CAD build for the part. Positions are in the model's coordinates, mm. Give positions to 0.01 mm unless a question says otherwise; leave off trailing zeros. Loops run counter-clockwise (first coordinate to the right, second up) from the corner with the lowest first, then second, coordinate; pieces in that order, holes last.
```python
from build123d import *

# Parameters (mm, degrees)
F0_R     = 15.875
F0_R_2   = 9.525
F1_DEPTH = 25.4
F2_DEPTH = 25.4


with BuildPart() as f1:
    # F0 (on Top) → F1 (new body)
    with BuildSketch(Plane.XY):
        with BuildLine():
            ThreePointArc((5.357812, -28.068211), (22.018516, -18.21306), (28.575, 0))
            ThreePointArc((28.575, 0), (22.018516, 18.21306), (5.357812, 28.068211))
            ThreePointArc((5.357812, 28.068211), (-28.575, 0), (5.357812, -28.068211))
        make_face()
        Circle(F0_R, mode=Mode.SUBTRACT)
        with BuildLine():
            ThreePointArc((69.85, 0), (65.479011, 12.14204), (54.371875, 18.712141))
            ThreePointArc((54.371875, 18.712141), (31.75, 0), (54.371875, -18.712141))
            ThreePointArc((54.371875, -18.712141), (65.479011, -12.14204), (69.85, 0))
        make_face()
        with Locations((50.8, 0)):
            Circle(F0_R_2, mode=Mode.SUBTRACT)
        with BuildLine():
            ThreePointArc((5.357812, 28.068211), (22.018516, 18.21306), (28.575, 0))
            ThreePointArc((28.575, 0), (22.018516, -18.21306), (5.357812, -28.068211))
            Line((5.357813, -28.068211), (54.371875, -18.712141))
            ThreePointArc((54.371875, -18.712141), (31.75, 0), (54.371875, 18.712141))
            Line((54.371875, 18.712141), (5.357812, 28.068211))
        make_face()
    extrude(amount=-F1_DEPTH)

    # F0 (on Top) → F2 (join)
    with BuildSketch(Plane.XY):
        with BuildLine():
            ThreePointArc((5.357812, -28.068211), (22.018516, -18.21306), (28.575, 0))
            ThreePointArc((28.575, 0), (22.018516, 18.21306), (5.357812, 28.068211))
            ThreePointArc((5.357812, 28.068211), (-28.575, 0), (5.357812, -28.068211))
        make_face()
        Circle(F0_R, mode=Mode.SUBTRACT)
    extrude(amount=F2_DEPTH)


solid = f1.part
```
1. Saw through at C-C, the plane y = -17. List the corners of the cut face in (x, z).
Responses:
outline: (-22.97, -25.4) - (59.4, -25.4) - (59.4, 0) - (22.97, 0) - (22.97, 25.4) - (-22.97, 25.4) - close
2. Probe line 1 along Y through (x, z) = (0, 7) (3 decimals); line 2 along Z through (x, y) = (63, -7); line 3 along Y through (x, z) = (-7.5, 23.5). List the from-to ranges inside material, lowest first.
Responses:
line 1: y = -28.575 to -15.875, 15.875 to 28.575
line 2: z = -25.4 to 0
line 3: y = -27.57 to -13.99, 13.99 to 27.57
3. Saw through at A-A, the plane x = 0. List the corners of the cut face in (y, z) (3 decimals), and give its area (3 significant figures).
Responses:
outline: (-28.575, -25.4) - (-15.875, -25.4) - (-15.875, 25.4) - (-28.575, 25.4) - close; (15.875, -25.4) - (28.575, -25.4) - (28.575, 25.4) - (15.875, 25.4) - close
area: 1,290 mm2
4. Saw through at B-B, the plane z = 13.5. List the corners of the cut face in (x, y) (3 decimals), and give its area (3 significant figures).
Responses:
outline: (5.358, -28.068) arc R28.575 ccw to (28.575, 0) arc R28.575 ccw to (5.358, 28.068) arc R28.575 ccw (long way) to start; hole circle Ø31.75 at (0, 0)
area: 1,770 mm2
5. Drop flat-ended pins along their axis: pin 1 (10 mm diameter, centred on x = 16, z = -8, fed in from +Y); pin 2 (3 mm diameter, centred on y = 10, z = -4, fed in from +X); pin 3 (3 mm diameter, centred on y = 16.5, z = -10, fed in from +X); pin 4 (11.5 mm diameter, centred on x = 50.8, y = 0, fed in from -Z). Give the stop position or say it passes through.
Responses:
pin 1: stops at y = 26.99
pin 2: stops at x = 67.85
pin 3: stops at x = 62.54
pin 4: passes through
6. Saw through at D-D, the plane x = 45. List the corners of the cut face in (y, z), and give its area (3 significant figures).
Responses:
outline: (-20.5, -25.4) - (-7.56, -25.4) - (-7.56, 0) - (-20.5, 0) - close; (7.56, -25.4) - (20.5, -25.4) - (20.5, 0) - (7.56, 0) - close
area: 658 mm2
7. Pull direction X, two halves, no side cores. Call faces 1 (the face through (29.522, -23.456, -12.522)), 2 (the face through (37, 0, 0)), 3 (the face through (59.6, -3.65, -12.52)): released by +X, released by -X, zero draft, split by the parting line, or undercut.
Responses:
face 1: released by +X
face 2: zero draft
face 3: undercut
